CAD build for the part. Positions are in the model's coordinates, mm. Face numbers are marked on the shaded views. A direction names the side the tool comes from. Coordinates: 2 decimals unless noted, no trailing zeros. Loops run counter-clockwise (first coordinate to the right, second up) from the corner with the lowest first, then second, coordinate; pieces in that order, holes last. Notation, with made-up numbers: (89, -23.5) -> (128, -23.5) arc R18 ccw to (128, -1.5) -> close; hole circle Ø5 at (17.25, 5.25). An arc over 180 degrees is marked (long way). Answer as a JSON object with one key per item and string values. Group by question number.
from build123d import *

# Parameters (mm, degrees)
BOSS_EXTRUDE1_DEPTH               = 12.7
F_1_4_CLEARANCE_HOLE1_D           = 6.7564
F_1_4_CLEARANCE_HOLE1_CSINK_D     = 8.0264
F_1_4_CLEARANCE_HOLE1_CSINK_ANGLE = 90
BOSS_EXTRUDE2_START               = -25.4
BOSS_EXTRUDE2_DEPTH               = 25.4
F_10_CLEARANCE_HOLE1_D            = 5.1054
F_10_CLEARANCE_HOLE1_CSINK_D      = 6.3754
F_10_CLEARANCE_HOLE1_CSINK_ANGLE  = 90
CUT_EXTRUDE1_START                = -7.62
SKETCH13_R                        = 4.445
CUT_EXTRUDE1_DEPTH                = 25.4


with BuildPart() as part:
    # Sketch1 → Boss-Extrude1 (new, symmetric)
    with BuildSketch(Plane.XY):
        with BuildLine():
            Line((-50.700684167, 47.625), (-66.575684167, 47.625))
            Line((-66.575684167, 47.625), (-66.575684167, 34.925))
            Line((-66.575684167, 34.925), (-53.577595831, 34.925))
            ThreePointArc((-53.577595831, 34.925), (0, -5.08), (53.577595831, 34.925))
            Line((53.577595831, 34.925), (66.575684167, 34.925))
            Line((66.575684167, 34.925), (66.575684167, 47.625))
            Line((66.575684167, 47.625), (50.700684167, 47.625))
            ThreePointArc((50.700684167, 47.625), (0, 0), (-50.700684167, 47.625))
        make_face()
    extrude(amount=BOSS_EXTRUDE1_DEPTH, both=True)

    # 1/4 Clearance Hole1 (through all)
    with Locations(Plane(origin=(0, 34.925, 0), x_dir=(-1, 0, 0), z_dir=(0, -1, 0))):
        with Locations((60.076639999, 0), (-60.076639999, 0)):
            CounterSinkHole(F_1_4_CLEARANCE_HOLE1_D / 2, F_1_4_CLEARANCE_HOLE1_CSINK_D / 2, counter_sink_angle=F_1_4_CLEARANCE_HOLE1_CSINK_ANGLE)

    # Sketch5 → Boss-Extrude2 (add)
    with BuildSketch(Plane(origin=(0, 0, -12.7), x_dir=(-1, 0, 0), z_dir=(0, 0, -1)).offset(BOSS_EXTRUDE2_START)):
        with BuildLine():
            Line((-31.75, -7.883822155), (31.75, -7.883822155))
            Line((31.75, -7.883822155), (31.75, 4.816177845))
            ThreePointArc((31.75, 4.816177845), (0, -5.08), (-31.75, 4.816177845))
            Line((-31.75, 4.816177845), (-31.75, -7.883822155))
        make_face()
    extrude(amount=BOSS_EXTRUDE2_DEPTH)

    # #10 Clearance Hole1 (through all)
    with Locations(Plane(origin=(0, -7.883822155, 0), x_dir=(-1, 0, 0), z_dir=(0, -1, 0))):
        with Locations((24.13, 0), (-24.13, 0)):
            CounterSinkHole(F_10_CLEARANCE_HOLE1_D / 2, F_10_CLEARANCE_HOLE1_CSINK_D / 2, counter_sink_angle=F_10_CLEARANCE_HOLE1_CSINK_ANGLE)

    # Sketch13 → Cut-Extrude1 (cut)
    with BuildSketch(Plane.XZ.offset(7.883822155).offset(CUT_EXTRUDE1_START)):
        with Locations(Location((-24.13, 0, 0), (0, 0, 270))):
            Circle(SKETCH13_R)
        with Locations(Location((24.13, 0, 0), (0, 0, 270))):
            Circle(SKETCH13_R)
    extrude(amount=-CUT_EXTRUDE1_DEPTH, mode=Mode.SUBTRACT)


solid = part.part
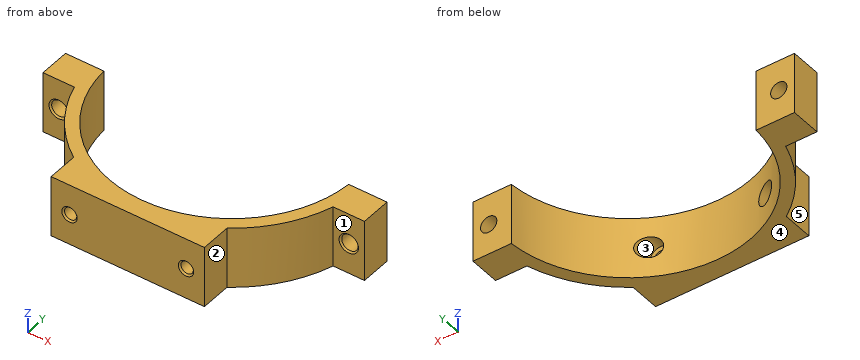
Item 1: Band-saw the part on C-C, the plane x = 24.13. List the corners of the cut face in (y, z) (3 decimals), and give its area (3 significant figures).
Item 2: Drill centre lines: L1, parallel to Z at x = -24.13, y = -3.75; L2, parallel to X at y = 40, z = -5.5; L3, parallel to Z at x = -24.13, y = 4 (3 decimals). Where is each one in solid material? Low to high.
Item 3: Pull direction X, two halves, no side cores. Call the marked faces 1, 2 and 3: +X half, -X half, draft (parallel to the pull), parting line (faces both ways), or undercut.
Item 4: Band-saw the part on D-D, the plane z = 0. Count the separate pieces of the cut face and the enclosed holes in it, and give its area (3 significant figures).
Item 5: Band-saw the part on A-A, the plane y = 21. List the corners of the cut face in (x, z), and give its area (3 significant figures).
Item 6: 3-axis set-ups, long thin cutter, end or side, ignore diameter. For the marked faces 4 and 5: which of +Z, -Z, +X, -X, +Y, -Y reach the whole face in a straight line?
Item 7: Band-saw the part on B-B, the plane z = -6.25. List the corners of the cut face in (x, y) (3 decimals).
Item 8: Flat gauge pins, fed straight in: P1, Ø4, axis at y = 0, z = 1.5, coming from the -X side; P2, Ø1, axis at x = 32.5, z = -5, coming from the +Y side; P3, Ø4.5, axis at x = 24.5, z = 0, coming from the +Y side; P4, Ø7, axis at x = 24.13, z = 0, coming from the -Y side. Where does each tip first touch, or does it go through?
Reply:
{
 "1": {"outline": "(-7.884, -12.7) -> (6.097, -12.7) -> (6.097, -4.445) -> (-0.264, -4.445) -> (-0.264, -2.553) -> (-7.249, -2.553) -> (-7.884, -3.188) -> close; (-7.884, 3.188) -> (-7.249, 2.553) -> (-0.264, 2.553) -> (-0.264, 4.445) -> (6.097, 4.445) -> (6.097, 12.7) -> (-7.884, 12.7) -> close", "area": "259 mm²"},
 "2": {"L1": "-12.7 to -2.55, 2.55 to 12.7", "L2": "-66.58 to -49.64, 49.64 to 66.58", "L3": "-12.7 to -4.445, 4.445 to 12.7"},
 "3": {"face 1": "draft", "face 2": "+X half", "face 3": "undercut"},
 "4": {"separate pieces": "5", "enclosed holes": "0", "area": "1,130 mm²"},
 "5": {"outline": "(-47.27, -12.7) -> (-41.14, -12.7) -> (-41.14, 12.7) -> (-47.27, 12.7) -> close; (41.14, -12.7) -> (47.27, -12.7) -> (47.27, 12.7) -> (41.14, 12.7) -> close", "area": "311 mm²"},
 "6": {"face 4": "-Z, +X, -X, +Y, -Y", "face 5": "+Z, -Z, -X, -Y"},
 "7": {"outline": "(-66.576, 34.925) -> (-53.578, 34.925) arc R55.88 ccw to (-31.75, 4.816) -> (-31.75, -7.884) -> (31.75, -7.884) -> (31.75, 4.816) arc R55.88 ccw to (53.578, 34.925) -> (66.576, 34.925) -> (66.576, 47.625) -> (50.701, 47.625) arc R50.8 cw to (-50.701, 47.625) -> (-66.576, 47.625) -> close"},
 "8": {"P1": "x = -31.75", "P2": "y = 12.18", "P3": "y = -0.26", "P4": "y = -7.88"}
}
